```python
from build123d import *
from build123d.topology import SkipClean

# Parameters (mm, degrees)
BOSS_EXTRUDE1_DEPTH = 5
CIRPATTERN1_COUNT   = 3
BOSS_EXTRUDE2_START = 6
BOSS_EXTRUDE2_DEPTH = 14
FILLET1_R           = 4
FILLET2_R           = 0.5
SKETCH15_W          = 2
SKETCH15_H          = 8
CUT_EXTRUDE1_DEPTH  = 120.910149393
CIRPATTERN2_COUNT   = 3


with BuildPart() as part:
    # Sketch8 → Revolve1 (revolve)
    with BuildSketch(Plane.XY, mode=Mode.PRIVATE) as revolve1_sk:
        with BuildLine():
            Line((13, 32), (14, 32))
            Line((14, 32), (14, 22))
            Line((14, 22), (22.5, 22))
            Line((22.5, 22), (22.5, 20))
            Line((22.5, 20), (24.5, 20))
            Line((24.5, 20), (24.5, 6))
            Line((24.5, 6), (0, 6))
            Line((0, 6), (0, 112))
            Line((0, 112), (11, 112))
            ThreePointArc((11, 112), (12.414213562, 111.414213562), (13, 110))
            Line((13, 110), (13, 32))
        make_face()
    revolve(revolve1_sk.sketch.rotate(Axis((0, 22, 0), (0, 1, 0)), 90), axis=Axis((0, 22, 0), (0, 1, 0)))

    # Sketch9 → Boss-Extrude1 (add, symmetric)
    with BuildSketch(Plane.XY):
        with BuildLine():
            Line((13, 32), (14, 32))
            Line((14, 32), (14, 22))
            Line((14, 22), (0, 22))
            Line((0, 22), (0, 112))
            Line((0, 112), (11, 112))
            ThreePointArc((11, 112), (12.414213562, 111.414213562), (13, 110))
            Line((13, 110), (13, 32))
        make_face()
    boss_extrude1 = extrude(amount=BOSS_EXTRUDE1_DEPTH, both=True)

    # CirPattern1: Boss-Extrude1 ×3 about axis
    cirpattern1_axis = Axis((0, 0, 0), (0, 1, 0))
    for i in range(1, CIRPATTERN1_COUNT):
        add(boss_extrude1.rotate(cirpattern1_axis, i * 360 / CIRPATTERN1_COUNT))

    # Sketch13 → Boss-Extrude2 (add)
    with BuildSketch(Plane(origin=(0, 0, 0), x_dir=(1, 0, 0), z_dir=(0, 1, 0)).offset(BOSS_EXTRUDE2_START)):
        with BuildLine():
            Line((-24.473491319, -1.139395744), (-31.105691219, -4.968498142))
            ThreePointArc((-31.105691219, -4.968498142), (-31.258439449, -3.893579744), (-31.374053012, -2.814035819))
            Line((-31.374053012, -2.814035819), (-24.472006051, 1.170862852))
            ThreePointArc((-24.472006051, 1.170862852), (-24.499994937, 0.015751071), (-24.473491319, -1.139395744))
        make_face()
        with BuildLine():
            Line((13.223491319, -20.624967329), (19.855691219, -24.454069727))
            ThreePointArc((19.855691219, -24.454069727), (19.001158695, -25.123812773), (18.124053012, -25.763709019))
            Line((18.124053012, -25.763709019), (11.222006051, -21.778810348))
            ThreePointArc((11.222006051, -21.778810348), (12.236356641, -21.225493543), (13.223491319, -20.624967329))
        make_face()
        with BuildLine():
            Line((24.473491319, 1.139395744), (31.105691219, 4.968498142))
            ThreePointArc((31.105691219, 4.968498142), (31.258439449, 3.893579744), (31.374053012, 2.814035819))
            Line((31.374053012, 2.814035819), (24.472006051, -1.170862852))
            ThreePointArc((24.472006051, -1.170862852), (24.499994937, -0.015751071), (24.473491319, 1.139395744))
        make_face()
        with BuildLine():
            Line((11.25, 21.764363074), (11.25, 29.422567869))
            ThreePointArc((11.25, 29.422567869), (12.257280754, 29.017392517), (13.25, 28.577744838))
            Line((13.25, 28.577744838), (13.25, 20.607947496))
            ThreePointArc((13.25, 20.607947496), (12.263638296, 21.209742473), (11.25, 21.764363074))
        make_face()
        with BuildLine():
            Line((-13.223491319, 20.624967329), (-19.855691219, 24.454069727))
            ThreePointArc((-19.855691219, 24.454069727), (-19.001158695, 25.123812773), (-18.124053012, 25.763709019))
            Line((-18.124053012, 25.763709019), (-11.222006051, 21.778810348))
            ThreePointArc((-11.222006051, 21.778810348), (-12.236356641, 21.225493543), (-13.223491319, 20.624967329))
        make_face()
        with BuildLine():
            Line((-11.25, -21.764363074), (-11.25, -29.422567869))
            ThreePointArc((-11.25, -29.422567869), (-12.257280754, -29.017392517), (-13.25, -28.577744838))
            Line((-13.25, -28.577744838), (-13.25, -20.607947496))
            ThreePointArc((-13.25, -20.607947496), (-12.263638296, -21.209742473), (-11.25, -21.764363074))
        make_face()
    extrude(amount=BOSS_EXTRUDE2_DEPTH)

    # Fillet1
    fillet1_edges = [part.edges().sort_by_distance(p)[0] for p in [
        (-24.473491319, 13, 1.139395744),
        (-24.472006051, 13, -1.170862852),
        (-11.25, 13, 21.764363074),
        (-13.25, 13, 20.607947496),
        (-13.223491319, 13, -20.624967329),
        (-11.222006051, 13, -21.778810348),
        (11.25, 13, -21.764363074),
        (13.25, 13, -20.607947496),
        (24.473491319, 13, -1.139395744),
        (24.472006051, 13, 1.170862852),
        (13.223491319, 13, 20.624967329),
        (11.222006051, 13, 21.778810348),
    ]]
    fillet(fillet1_edges, radius=FILLET1_R)

    # Fillet2
    fillet2_edges = [part.edges().sort_by_distance(p)[0] for p in [
        (-31.374053012, 13, 2.814035819),
        (-31.105691219, 13, 4.968498142),
        (-13.25, 13, 28.577744838),
        (-11.25, 13, 29.422567869),
        (-18.124053012, 13, -25.763709019),
        (-19.855691219, 13, -24.454069727),
        (13.25, 13, -28.577744838),
        (11.25, 13, -29.422567869),
        (31.374053012, 13, -2.814035819),
        (31.105691219, 13, -4.968498142),
        (18.124053012, 13, 25.763709019),
        (19.855691219, 13, 24.454069727),
    ]]
    fillet(fillet2_edges, radius=FILLET2_R)

    # Sketch15 → Cut-Extrude1 (cut, through all)
    with BuildSketch(Plane(origin=(0, 0, 0), x_dir=(1, 0, 0), z_dir=(0, 1, 0))):
        with Locations((14, 0)):
            Rectangle(SKETCH15_W, SKETCH15_H)
    cut_extrude1 = extrude(amount=CUT_EXTRUDE1_DEPTH, mode=Mode.SUBTRACT)

    # CirPattern2: Cut-Extrude1 ×3 about axis
    cirpattern2_axis = Axis((0, 0, 0), (0, 1, 0))
    for i in range(1, CIRPATTERN2_COUNT):
        add(cut_extrude1.rotate(cirpattern2_axis, i * 360 / CIRPATTERN2_COUNT), mode=Mode.SUBTRACT)

    # Sketch16 → Cut-Revolve1 (revolve, cut)
    with SkipClean():  # the faces are left unmerged after this step: merging them gives an invalid solid
        with BuildSketch(Plane.XY, mode=Mode.PRIVATE) as cut_revolve1_sk:
            Polygon((11, 6), (14, 9), (17, 6), align=None)
        revolve(cut_revolve1_sk.sketch.rotate(Axis((0, 0, 0), (0, 1, 0)), 257.102728972), axis=Axis((0, 0, 0), (0, 1, 0)), mode=Mode.SUBTRACT)


solid = part.part
```
Check sheet for the modelled part. Datum: model origin and axes. Units: mm. A direction names the side the tool comes from. Round coordinates to 2 decimals unless told otherwise and drop trailing zeros. Loops run counter-clockwise (first coordinate to the right, second up) from the corner with the lowest first, then second, coordinate; pieces in that order, holes last. Notation, with made-up numbers: M -23,-33 L 4,-33 A19 ccw 4,4 Z; hole C 7,-15 d1. An arc over 180 degrees is marked long. Answer as a JSON object with one key per item and string values.
1. Gauge pin test, flat ends, axial feed: P1, Ø0.5, axis at y = 26, z = 4.5, coming from the +X side; P2, Ø0.7, axis at x = 13.5, y = 25, coming from the +Z side; P3, Ø4, axis at y = 46.5, z = 8.5, coming from the +X side. Record the tip position at first contact, or that the pin passes through.
Reply:
{"P1": "stops at x = 14", "P2": "stops at z = 5", "P3": "stops at x = 11.26"}
2. Access from +Z, -Z, +X, -X, +Y, -Y to the whole of each face (thin tool, end or side, straight path). Record for faces 4 (the flat face through (-10.45, 72.19, -8.1)), 5 (the flat face through (15, 15, 0)), 6 (the flat face through (12.2, 72.2, -5)), 7 (the flat face through (-15.47, 12.9, -24.23)).
Reply:
{"face 4": "-X, +Y", "face 5": "+Y, -Y", "face 6": "-Z, +X, +Y", "face 7": "-Z, +Y, -Y"}
3. Mould release check, pull along X, two halves, no side actions. Record for faces 1 (the flat face through (-13.25, 13, 26)), 2 (the flat face through (-7.55, 14.64, 12.96)), 3 (the cylindrical face through (20.37, 12.9, -13.61)): pulls with the +X half, pulls with the -X half, needs draft (parallel to the pull), parting line crosses it, or undercut.
Reply:
{"face 1": "pulls with the -X half", "face 2": "undercut", "face 3": "pulls with the +X half"}
4. Scan lines: line 1 (Y direction, x = -24, z = -0.5); line 2 (Z direction, x = 14, y = 20.5); line 3 (Y direction, x = 16.5, z = -15). Record each from-to range of solid material in increasing order.
Reply:
{"line 1": "y = 6 to 20", "line 2": "z = -17.61 to -4, 4 to 17.61", "line 3": "y = 6 to 22"}
5. Section check A-A (y = 26). Record the boundary of the cut face in (x, z).
Reply:
{"outline": "M -11.33,-9.62 L -10.46,-10.12 L -9.96,-9.26 L -3.04,-13.26 L -3.54,-14.12 L -2.67,-14.62 L -2.21,-13.82 A14 ccw 13.08,-5 L 14,-5 L 14,-4 L 13,-4 L 13,4 L 14,4 L 14,5 L 13.08,5 A14 ccw -2.21,13.82 L -2.67,14.62 L -3.54,14.12 L -3.04,13.26 L -9.96,9.26 L -10.46,10.12 L -11.33,9.62 L -10.87,8.82 A14 ccw -10.87,-8.82 Z"}
6. Section check B-B (y = 62). Record the boundary of the cut face in (x, z).
Reply:
{"outline": "M -10.83,-8.76 L -2.17,-13.76 L -1.67,-12.89 A13 ccw 12,-5 L 13,-5 L 13,5 L 12,5 A13 ccw -1.67,12.89 L -2.17,13.76 L -10.83,8.76 L -10.33,7.89 A13 ccw -10.33,-7.89 Z"}
